Autodesk Inventor part; units mm, degrees
ref_plane "YZ Plane" through (0, 0, 0) normal (1, 0, 0) x (0, 1, 0)
ref_plane "XZ Plane" through (0, 0, 0) normal (0, 1, 0) x (-1, 0, 0)
ref_plane "XY Plane" through (0, 0, 0) normal (0, 0, 1) x (1, 0, 0)
ref_plane "Work Plane1" through (0, 0.5, 0) normal (0, 0, 1) x (1, 0, 0)
sketch "Sketch1" plane through (0, 0.5, 0) normal (0, 0, 1) x (1, 0, 0)
  arc A0 (-25.85, 13.75) -> (-27.85, 11.75) centre (-25.85, 11.75) ccw
  line L0 (-27.85, 11.75) -> (-27.85, -5.75)
  arc A1 (-27.85, -5.75) -> (-25.85, -7.75) centre (-25.85, -5.75) ccw
  line L1 (-25.85, -7.75) -> (-19.4, -7.75)
  arc A2 (-17.4, -9.75) -> (-19.4, -7.75) centre (-19.4, -9.75) ccw
  line L2 (-17.4, -9.75) -> (-17.4, -12.466667)
  arc A3 (-17.4, -12.466667) -> (-15.4, -14.466667) centre (-15.4, -12.466667) ccw
  line L3 (-15.4, -14.466667) -> (1.1, -14.466667)
  arc A4 (1.1, -14.466667) -> (3.1, -12.466667) centre (1.1, -12.466667) ccw
  line L4 (3.1, -12.466667) -> (3.1, -9.75)
  arc A5 (5.1, -7.75) -> (3.1, -9.75) centre (5.1, -9.75) ccw
  line L5 (5.1, -7.75) -> (24.95, -7.75)
  arc A6 (24.95, -7.75) -> (26.95, -5.75) centre (24.95, -5.75) ccw
  line L6 (26.95, -5.75) -> (26.95, 11.941667)
  arc A7 (26.95, 11.941667) -> (24.95, 13.941667) centre (24.95, 11.941667) ccw
  line L7 (24.95, 13.941667) -> (19.95, 13.941667)
  line L8 (19.95, 13.941667) -> (19.95, -5.75)
  line L9 (19.95, -5.75) -> (1.6, -5.75)
  line L10 (1.6, -5.75) -> (1.1, -12.466667)
  line L11 (1.1, -12.466667) -> (-13.9, -12.75)
  line L12 (-15.4, -12.75) -> (-15.4, -5.75)
  line L13 (-15.4, -5.75) -> (-20.85, -5.75)
  line L14 (-20.85, -5.75) -> (-20.85, 13.75)
  line L15 (-20.85, 13.75) -> (-25.85, 13.75)
  circle A8 centre (23.55, -1.25) radius 1.25
  circle A9 centre (-24.45, -1.25) radius 1.25
  circle A10 centre (-24.45, 8.25) radius 1.25
  circle A11 centre (23.55, 8.25) radius 1.25
  line L16 (-20.4, -5.75) -> (-20.4, -7.75)
  line L17 (-13.9, -12.75) -> (-15.4, -12.75)
  point P0 (0, -0.5)
sketch "Sketch1 outline for Extrusion1" plane through (0, 0.5, 0) normal (0, 0, 1) x (1, 0, 0)
  line L0 (-20.85, -5.75) -> (-20.85, 13.75)
  line L1 (-19.4, -7.75) -> (-20.85, -5.75)
  line L2 (-20.85, 13.75) -> (-25.85, 13.75)
  line L3 (-25.85, -7.75) -> (-19.4, -7.75)
  arc A0 (-25.85, 13.75) -> (-27.85, 11.75) centre (-25.85, 11.75) ccw
  arc A1 (-27.85, -5.75) -> (-25.85, -7.75) centre (-25.85, -5.75) ccw
  line L4 (-27.85, 11.75) -> (-27.85, -5.75)
  circle A2 centre (-24.45, -1.25) radius 1.25
  circle A3 centre (-24.45, 8.25) radius 1.25
extrude "Extrusion1" add sketch "Sketch1 outline for Extrusion1" along normal blind 5
ref_plane "Work Plane2" through (-25.85, 3.5, 0) normal (0, -1, 0) x (1, 0, 0)
sketch "Sketch3" plane through (-20.85, -7.25, 0) normal (1, 0, 0) x (0, 0, -1)
  line L0 (0, 19.5) -> (-5, 19.5)
  line L1 (0, 21.5) -> (-5, 21.5)
  line L2 (0, 21.5) -> (0, 19.5)
  arc A0 (0, 21.5) -> (-26.539944, 48.039944) centre (-26.539944, 21.5) ccw
  line L3 (-26.539944, 48.039944) -> (-35, 48.039944)
  line L4 (-35, 48.039944) -> (-35, 46.366043)
  line L5 (-35, 46.366043) -> (-28.232934, 46.005114)
  arc A1 (-5, 21.5) -> (-28.232934, 46.005114) centre (-29.539944, 21.5) ccw
  line L6 (-5, 2) -> (-5, 21.5)
  line L7 (0, 2) -> (0, 21.5)
  point P0 (0, 7.25)
  point P1 (-5, 0)
  point P2 (0, 0)
  dimension "d9" = 3
  dimension "d12" = 35
extrude "Extrusion2" add sketch "Sketch3" against normal blind 5 contours L1 A1 L5 L4 L3 A0
sketch "Sketch2" plane through (0, 0.5, 5) normal (0, 0, 1) x (1, 0, 0)
  circle A0 centre (-24.45, -1.25) radius 1.25
  circle A1 centre (-24.45, 8.25) radius 1.25
  point P0 (0, -0.5)
hole "Hole1" at (-24.45, -0.75, 5) at (-24.45, 8.75, 5) direction (0, 0, -1) diameter 3.2 end through all counterbore diameter 6.5 counterbore depth 1
mirror "Mirror1" about plane through (-25.85, 3.5, 0) normal (0, -1, 0) of "Extrusion2"
properties part number "leg"
Could you check a few things on this model? Use its own coordinates, in mm. A direction names the side the tool comes from. Round coordinates to 2 decimals unless told otherwise and drop trailing zeros. Write each loop counter-clockwise with the first axis right and the second up, starting at its lowest first coordinate (ties: lowest second). Pieces come first, ordered by that corner, then holes. Notation, with made-up numbers: (64.5, 83.5) - (97.5, 83.5) arc R20 cw to (97.5, 107.5) - close; hole circle Ø11 at (38.25, 31). An arc over 180 degrees is marked (long way). Use a Markdown table: item, result.
Q1. I want a section at B-B (x = -24.45). List the corners of the cut face in (y, z) for me, plus the area to 3 significant figures.
Output values:
| item | result |
|---|---|
| outline | (-33.79, 26.54) arc R26.54 ccw to (-7.25, 0) - (-2.35, 0) - (-2.35, 4) - (-4, 4) - (-4, 5) - (-7.25, 5) arc R24.54 cw to (-31.76, 28.23) - (-32.12, 35) - (-33.79, 35) - close; (0.85, 0) - (7.15, 0) - (7.15, 4) - (5.5, 4) - (5.5, 5) - (2.5, 5) - (2.5, 4) - (0.85, 4) - close; (10.35, 0) - (14.25, 0) arc R26.54 ccw to (40.79, 26.54) - (40.79, 35) - (39.12, 35) - (38.76, 28.23) arc R24.54 cw to (14.25, 5) - (12, 5) - (12, 4) - (10.35, 4) - close |
| area | 408 mm2 |
Q2. For pin 1 (1.5 mm diameter, centred on y = -26, z = 13, fed in from -X); pin 2 (4 mm diameter, centred on x = -25.5, z = 20, fed in from -Y); pin 3 (4 mm diameter, centred on x = -24.5, y = 2.5, fed in from +Z), each with a flat end and sliding along its axis, tell me the tip position at first contact or that it passes through.
Output values:
| item | result |
|---|---|
| pin 1 | x = -25.85 |
| pin 2 | y = -33.4 |
| pin 3 | z = 5 |
Q3. Thinking about a two-plate mould opening in Y: for faces 5 (the flat face through (-23, -33.79, 31)), 6 (the cylindrical face through (-23.32, -24.32, 11.91)), 7 (the flat face through (-20.85, -24, 11)), which applies, released by +Y, released by -Y, zero draft, split by the parting line, or undercut?
Output values:
| item | result |
|---|---|
| face 5 | released by -Y |
| face 6 | undercut |
| face 7 | zero draft |
Q4. For faces 1 (the flat face through (-20, -7.25, 2)), 2 (the cylindrical face through (-27.672, -0.327, 4.493)), 3 (the flat face through (-25.85, 32, 11)), 4 (the flat face through (-20.85, 21.1, 5.8)), which set-ups out of +Z, -Z, +X, -X, +Y, -Y let a thin tool reach every point of the face, with its end or its side?
Output values:
| item | result |
|---|---|
| face 1 | +Z, -Z, +X, -Y |
| face 2 | +Z |
| face 3 | +Z, -Z, -X, +Y |
| face 4 | +Z, -Z, +X, +Y |
Q5. I want a section at C-C (z = 12). List the corners of the cut face in (x, y) for me, plus the area to 3 significant figures.
Output values:
| item | result |
|---|---|
| outline | (-25.85, -29.45) - (-20.85, -29.45) - (-20.85, -24.41) - (-25.85, -24.41) - close; (-25.85, 31.41) - (-20.85, 31.41) - (-20.85, 36.45) - (-25.85, 36.45) - close |
| area | 50.4 mm2 |
Q6. I want a section at D-D (z = 6). List the corners of the cut face in (x, y) for me, plus the area to 3 significant figures.
Output values:
| item | result |
|---|---|
| outline | (-25.85, -24.06) - (-20.85, -24.06) - (-20.85, -14.18) - (-25.85, -14.18) - close; (-25.85, 21.18) - (-20.85, 21.18) - (-20.85, 31.06) - (-25.85, 31.06) - close |
| area | 98.7 mm2 |
Q7. I want a section at A-A (y = 8.75). List the corners of the cut face in (x, z) for me, plus the area to 3 significant figures.
Output values:
| item | result |
|---|---|
| outline | (-27.85, 0) - (-26.05, 0) - (-26.05, 4) - (-27.7, 4) - (-27.7, 5) - (-27.85, 5) - close; (-22.85, 0) - (-20.85, 0) - (-20.85, 5) - (-21.2, 5) - (-21.2, 4) - (-22.85, 4) - close |
| area | 15.7 mm2 |
Q8. Please list where these lines run through material, in increasing order: L1, parallel to Y at x = -24.45, z = 4.7; L2, parallel to X at y = -0.75, z = 2.5; L3, parallel to X at y = 8.75, z = 4.8.
Output values:
| item | result |
|---|---|
| L1 | -22.33 to -4, 2.5 to 5.5, 12 to 29.33 |
| L2 | -27.85 to -26.05, -22.85 to -20.85 |
| L3 | -27.85 to -27.7, -21.2 to -20.85 |
